from build123d import *

# Parameters (mm, degrees)
F0_W     = 47.5
F0_H     = 18
F1_DEPTH = 5
F3_R     = 1.75
F4_DEPTH = 7.5


with BuildPart() as f1:
    # F0 (on Front) → F1 (new body)
    with BuildSketch(Plane.XZ):
        Rectangle(F0_W, F0_H)
        with BuildLine():
            ThreePointArc((1.396902, 1), (0, -0.396902), (-1.396902, 1))
            Line((-1.396902, 1), (-1.396902, 6))
            ThreePointArc((-1.396902, 6), (0, 7.396902), (1.396902, 6))
            Line((1.396902, 6), (1.396902, 1))
        make_face(mode=Mode.SUBTRACT)
    extrude(amount=F1_DEPTH)

    # F3 (on Right) → F4 (join, symmetric)
    with BuildSketch(Plane.YZ):
        with BuildLine():
            ThreePointArc((-2.5, -9), (-4.267767, -9.732233), (-5, -11.5))
            ThreePointArc((-5, -11.5), (-2.5, -14), (0, -11.5))
            ThreePointArc((0, -11.5), (-0.732233, -9.732233), (-2.5, -9))
        make_face()
        with Locations((-2.5, -11.5)):
            Circle(F3_R, mode=Mode.SUBTRACT)
        with BuildLine():
            ThreePointArc((-2.5, -9), (-0.732233, -9.732233), (0, -11.5))
            Line((0, -11.5), (0, -9))
            Line((0, -9), (-2.5, -9))
        make_face()
        with BuildLine():
            Line((-5, -9), (-5, -11.5))
            ThreePointArc((-5, -11.5), (-4.267767, -9.732233), (-2.5, -9))
            Line((-2.5, -9), (-5, -9))
        make_face()
    extrude(amount=F4_DEPTH, both=True)


solid = f1.part
Build history of the part. All positions in model axes, mm. A direction names the side the tool comes from. Give positions to 0.01 mm unless a question says otherwise; leave off trailing zeros. Order: outer loops, then holes, each group sorted by start corner. A loop starts at its lowest first (then second) coordinate and runs counter-clockwise, first axis right, second up. Notation, with made-up numbers: M 75.25,-33.75 L 83.25,-33.75 A25 ccw 83.25,-5.75 Z; hole C 83.25,-16 d4. An arc over 180 degrees is marked long. Use one line per item in the form item = value.
Q1. Pin check, flat tip, straight feed: P1, Ø2.5, axis at x = -12, y = -3.5, coming from the -Z side. Stop position of the tip, or through.
Conclusion:
P1 = -9
Q2. Slice it at A-A, the plane y = -2.5. Write the cut outline in (x, z), and give its area (3 significant figures).
Conclusion:
outline = M -23.75,-9 L -7.5,-9 L -7.5,-9.75 L 7.5,-9.75 L 7.5,-9 L 23.75,-9 L 23.75,9 L -23.75,9 Z; M -7.5,-14 L 7.5,-14 L 7.5,-13.25 L -7.5,-13.25 Z; hole M -1.4,1 A1.4 ccw 1.4,1 L 1.4,6 A1.4 ccw -1.4,6 Z
area = 857 mm2
Q3. Slice it at C-C, the plane z = 3.75. Write the cut outline in (x, y).
Conclusion:
outline = M -23.75,-5 L -1.4,-5 L -1.4,0 L -23.75,0 Z; M 1.4,-5 L 23.75,-5 L 23.75,0 L 1.4,0 Z
Q4. Which spindle directions (+Z, -Z, +X, -X, +Y, -Y) get a long thin tool onto all of the face, cutting with end or side? Do faces 4 (the cylindrical face through (0.031, -2.465, -0.397)), 5 (the flat face through (16, -2, -9)), 6 (the flat face through (-7.5, -4, -10)). Say none if no direction does.
Conclusion:
face_4 = +Y, -Y
face_5 = -Z, +X, +Y, -Y
face_6 = -Z, -X, +Y, -Y
Q5. Slice it at D-D, the plane x = -7. Write the cut outline in (y, z).
Conclusion:
outline = M -5,-11.5 A2.5 ccw 0,-11.5 L 0,9 L -5,9 Z; hole C -2.5,-11.5 d3.5
Q6. Pull direction X, two halves, no side cores. Call faces 1 (the flat face through (0, -2, 9)), 2 (the flat face through (7.5, -4, -10)), 3 (the flat face through (-1.397, -2, 3)): released by +X, released by -X, zero draft, split by the parting line, or undercut.
Conclusion:
face_1 = zero draft
face_2 = released by +X
face_3 = undercut
Q7. Slice it at B-B, the plane x = 0. Write the cut outline in (y, z), and give its area (3 significant figures).
Conclusion:
outline = M -5,-11.5 A2.5 ccw 0,-11.5 L 0,-0.4 L -5,-0.4 Z; M -5,7.4 L 0,7.4 L 0,9 L -5,9 Z; hole C -2.5,-11.5 d3.5
area = 63.7 mm2
Q8. Wall check: probe 1 along X at (y, z) = (-0.65, 4.75); probe 2 along Z at (x, y) = (-1.5, -2.5); probe 3 along Z at (x, y) = (-1, -2.5). Give the ranges that are in metal, low to high.
Conclusion:
probe_1 = -23.75 to -1.4, 1.4 to 23.75
probe_2 = -14 to -13.25, -9.75 to 9
probe_3 = -14 to -13.25, -9.75 to 0.02, 6.98 to 9
